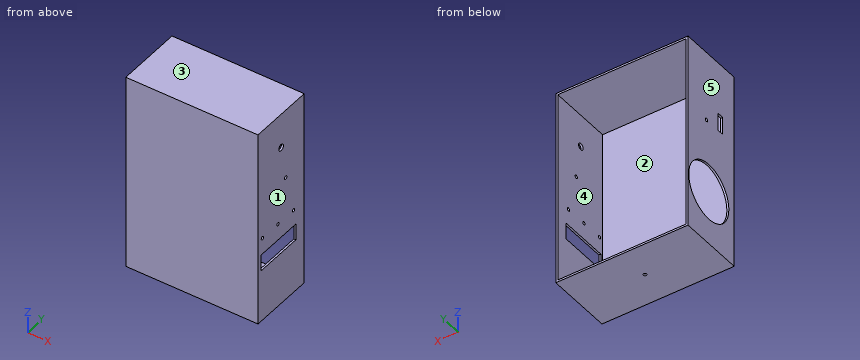
```python
from build123d import *

# Parameters (mm, degrees)
ESBO_O1_W                = 200
ESBO_O1_H                = 100
RESSALTO_EXTRUS_O1_DEPTH = 150
ESBO_O2_W                = 194
ESBO_O2_H                = 294
CORTE_EXTRUS_O1_DEPTH    = 97
ESBO_O5_R                = 5
CORTE_EXTRUS_O4_DEPTH    = 10
ESBO_O7_R                = 2.5
CORTE_EXTRUS_O6_DEPTH    = 10
ESBO_O8_W                = 27
ESBO_O8_H                = 10
CORTE_EXTRUS_O9_DEPTH    = 10
ESBO_O11_R               = 2.5
CORTE_EXTRUS_O12_DEPTH   = 201
ESBO_O12_R               = 2.5
ESBO_O12_W               = 25
ESBO_O12_H               = 75
CORTE_EXTRUS_O13_DEPTH   = 10
ESBO_O13_R               = 43.358301647
CORTE_EXTRUS_O14_DEPTH   = 10


with BuildPart() as part:
    # Esboço1 → Ressalto-extrusão1 (new body, symmetric)
    with BuildSketch(Plane.XY):
        Rectangle(ESBO_O1_W, ESBO_O1_H)
    extrude(amount=RESSALTO_EXTRUS_O1_DEPTH, both=True)

    # Esboço2 → Corte-extrusão1 (cut)
    with BuildSketch(Plane(origin=(0, 50, 0), x_dir=(1, 0, 0), z_dir=(0, 1, 0))):
        Rectangle(ESBO_O2_W, ESBO_O2_H)
    extrude(amount=-CORTE_EXTRUS_O1_DEPTH, mode=Mode.SUBTRACT)

    # Esboço5 → Corte-extrusão4 (cut)
    with BuildSketch(Plane(origin=(100, 0, 0), x_dir=(0, 0, -1), z_dir=(1, 0, 0))):
        with Locations((-97.256103524, 0)):
            Circle(ESBO_O5_R)
    extrude(amount=-CORTE_EXTRUS_O4_DEPTH, mode=Mode.SUBTRACT)

    # Esboço7 → Corte-extrusão6 (cut)
    with BuildSketch(Plane(origin=(0, 0, -150), x_dir=(-1, 0, 0), z_dir=(0, 0, -1))):
        Circle(ESBO_O7_R)
    extrude(amount=-CORTE_EXTRUS_O6_DEPTH, mode=Mode.SUBTRACT)

    # Esboço8 → Corte-extrusão9 (cut)
    with BuildSketch(Plane.ZY.offset(100)):
        with Locations((56.5, -20)):
            Rectangle(ESBO_O8_W, ESBO_O8_H)
    extrude(amount=-CORTE_EXTRUS_O9_DEPTH, mode=Mode.SUBTRACT)

    # Esboço11 → Corte-extrusão12 (cut, through all)
    with BuildSketch(Plane.ZY.offset(100)):
        with Locations((43, 10)):
            Circle(ESBO_O11_R)
    extrude(amount=-CORTE_EXTRUS_O12_DEPTH, mode=Mode.SUBTRACT)

    # Esboço12 → Corte-extrusão13 (cut)
    with BuildSketch(Plane(origin=(100, 0, 0), x_dir=(0, 0, -1), z_dir=(1, 0, 0))):
        with Locations((20, 27)):
            Circle(ESBO_O12_R)
        with Locations((20, -6.75)):
            Circle(ESBO_O12_R)
        with Locations((20, -40.5)):
            Circle(ESBO_O12_R)
        with Locations((57.5, -5.5)):
            Rectangle(ESBO_O12_W, ESBO_O12_H)
    extrude(amount=-CORTE_EXTRUS_O13_DEPTH, mode=Mode.SUBTRACT)

    # Esboço13 → Corte-extrusão14 (cut)
    with BuildSketch(Plane.ZY.offset(100)):
        with Locations((-67.620059567, 5)):
            Circle(ESBO_O13_R)
    extrude(amount=-CORTE_EXTRUS_O14_DEPTH, mode=Mode.SUBTRACT)


solid = part.part
```
Design review of the part built by this model. Coordinates are the model's own, in mm. Face numbers are marked on the shaded views. A direction names the side the tool comes from. Coordinates: 2 decimals unless noted, no trailing zeros. Order: outer loops, then holes, each group sorted by start corner. A loop starts at its lowest first (then second) coordinate and runs counter-clockwise, first axis right, second up.
1) Take a section at D-D, the plane z = -124. Give the boundary of the cut face in (x, y).
2) Wall thickness on line 1 along Y through (x, z) = (98, -20); line 2 along X through (y, z) = (11, 52); line 3 along Y through (x, z) = (98, 43): over which ranges is each line inside the solid? List them lowest first.
3) Take a section at B-B, the plane z = -78. Give the boundary of the cut face in (x, y).
4) Take a section at A-A, the plane y = -30. Give the boundary of the cut face in (x, z).
5) Take a section at C-C, the plane x = -40. Give the boundary of the cut face in (y, z), and give its area (3 significant figures).
6) Clearance check with flat-ended pins moving along their axes: pin 1 (1.5 mm diameter, centred on x = -11, z = 115, fed in from +Y); pin 2 (4 mm diameter, centred on y = -1, z = -34.5, fed in from -X). State where each tip first meets the part, or that it passes through.
7) Mouldability with a two-part tool opening along X and no side actions: class the marked faces 1, 2 and 3 as +X half, -X half, draft (parallel to the pull), parting line (faces both ways), or undercut.
8) For the marked faces 4 and 5, list the 3-axis set-ups (+Z, -Z, +X, -X, +Y, -Y) from which the entire face can be reached by the end or side of a thin tool; tool diameter is ignored.
Returned:
1. outline: (-100, -50) - (100, -50) - (100, 50) - (97, 50) - (97, -47) - (-97, -47) - (-97, 50) - (-100, 50) - close
2. line 1: y = -50 to -43, -38 to -9.25, -4.25 to 24.5, 29.5 to 50
2. line 2: x = -100 to -97, 97 to 100
2. line 3: y = -50 to 7.5, 12.5 to 50
3. outline: (-100, -50) - (100, -50) - (100, 50) - (97, 50) - (97, -47) - (-97, -47) - (-97, -37.1) - (-100, -37.1) - close; (-100, 47.1) - (-97, 47.1) - (-97, 50) - (-100, 50) - close
4. outline: (-100, -150) - (100, -150) - (100, -70) - (97, -70) - (97, -147) - (-97, -147) - (-97, -93.21) - (-100, -93.21) - close; (-100, -42.03) - (-97, -42.03) - (-97, 147) - (97, 147) - (97, -45) - (100, -45) - (100, 150) - (-100, 150) - close
5. outline: (-50, -150) - (50, -150) - (50, -147) - (-47, -147) - (-47, 147) - (50, 147) - (50, 150) - (-50, 150) - close
5. area: 1,480 mm2
6. pin 1: stops at y = -47
6. pin 2: stops at x = 97
7. face 1: +X half
7. face 2: undercut
7. face 3: draft
8. face 4: +Y
8. face 5: +Z, -Z, -X, +Y, -Y
